```python
from build123d import *

# Parameters (mm, degrees)
BOSS_EXTRUDE1_DEPTH = 9.525
SKETCH2_R           = 2.2
M5_DRILL_DEPTH      = 9.525
SKETCH3_R           = 1.75
M4_DRILL_DEPTH      = 8


with BuildPart() as part:
    # Sketch1 → Boss-Extrude1 (new body)
    with BuildSketch(Plane.XY):
        with BuildLine():
            Line((-11, 3.5), (-11, -3.5))
            Line((-11, -3.5), (11, -3.5))
            Line((11, -3.5), (11, 3.5))
            ThreePointArc((11, 3.5), (0, 9.776932339), (-11, 3.5))
        make_face()
    extrude(amount=BOSS_EXTRUDE1_DEPTH)

    # Sketch2 → M5_DRILL (cut)
    with BuildSketch(Plane.XY.offset(9.525)):
        with Locations((0, 3.5)):
            Circle(SKETCH2_R)
    extrude(amount=-M5_DRILL_DEPTH, mode=Mode.SUBTRACT)

    # Sketch3 → M4_DRILL (cut)
    with BuildSketch(Plane.XZ.offset(3.5)):
        with Locations(Location((-6, 4.7625, 0), (0, 0, 270))):
            Circle(SKETCH3_R)
        with Locations(Location((6, 4.7625, 0), (0, 0, 90))):
            Circle(SKETCH3_R)
    extrude(amount=-M4_DRILL_DEPTH, mode=Mode.SUBTRACT)


solid = part.part
```
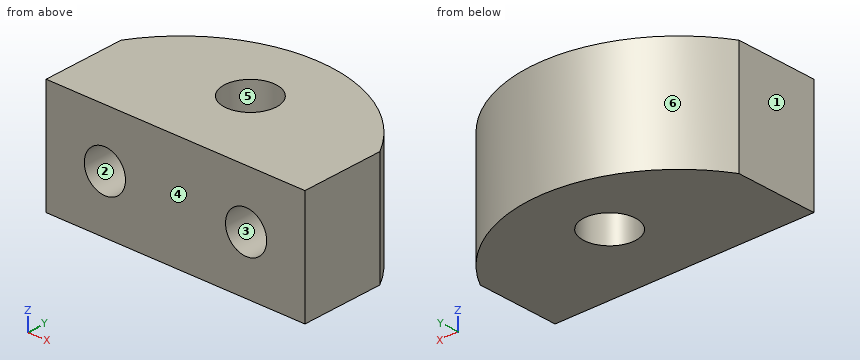
Could you check a few things on this model? Use its own coordinates, in mm. Face numbers are marked on the shaded views. A direction names the side the tool comes from. Coordinates: 2 decimals unless noted, no trailing zeros. Loops run counter-clockwise (first coordinate to the right, second up) from the corner with the lowest first, then second, coordinate; pieces in that order, holes last. Notation, with made-up numbers: M 54,-1.75 L 84,-1.75 A5 ccw 84,2.25 Z; hole C -7.5,5.5 d2. An arc over 180 degrees is marked long. Put each result on its own line as item: value. Start each with the question number.
(1) Suppose I cut it at C-C on z = 5.5. Please give me the cut outline in (x, y), then the cut area to 3 significant figures.
(2) For the marked faces 1 and 2, which set-ups out of +Z, -Z, +X, -X, +Y, -Y let a thin tool reach every point of the face, with its end or its side?
(3) Suppose I cut it at A-A on y = 2.5. Count the separate pieces of the cut face and the enclosed holes in it, then the cut area to 3 significant figures.
(4) I need wall thicknesses on line 1 (Y direction, x = 0, z = 7.5); line 2 (X direction, y = -2, z = 5.25); line 3 (Z direction, x = -5.5, y = 2.25) (3 decimals). Which ranges of each line are inside material? Lowest first, please. Write a range as from..to.
(5) Thinking about a two-plate mould opening in Y: for the marked faces 3, 4, 5 and 6, which applies, pulls with the +Y half, pulls with the -Y half, needs draft (parallel to the pull), parting line crosses it, or undercut?
(6) Suppose I cut it at B-B on x = 0. Please give me the cut outline in (y, z) (3 decimals), then the cut area to 3 significant figures.
(7) Will these pins go through, and if not, where does the flat tip stop? P1, Ø1.5, axis at x = -6.5, z = 1, coming from the +Y side; P2, Ø2, axis at x = 6, z = 4.76, coming from the -Y side.
Solutions:
1. outline: M -11,-3.5 L -7.59,-3.5 L -7.59,4.5 L -4.41,4.5 L -4.41,-3.5 L 4.41,-3.5 L 4.41,4.5 L 7.59,4.5 L 7.59,-3.5 L 11,-3.5 L 11,3.5 A12.78 ccw -11,3.5 Z; hole C 0,3.5 d4.4
1. area: 186 mm2
2. face 1: +Z, -Z, -X, +Y, -Y
2. face 2: -Y
3. separate pieces: 2
3. enclosed holes: 2
3. area: 153 mm2
4. line 1: y = -3.5..1.3, 5.7..9.78
4. line 2: x = -11..-7.68, -4.32..4.32, 7.68..11
4. line 3: z = 0..3.085, 6.44..9.525
5. face 3: needs draft
5. face 4: pulls with the -Y half
5. face 5: undercut
5. face 6: pulls with the +Y half
6. outline: M -3.5,0 L 1.3,0 L 1.3,9.525 L -3.5,9.525 Z; M 5.7,0 L 9.777,0 L 9.777,9.525 L 5.7,9.525 Z
6. area: 84.6 mm2
7. P1: stops at y = 8.41
7. P2: stops at y = 4.5
